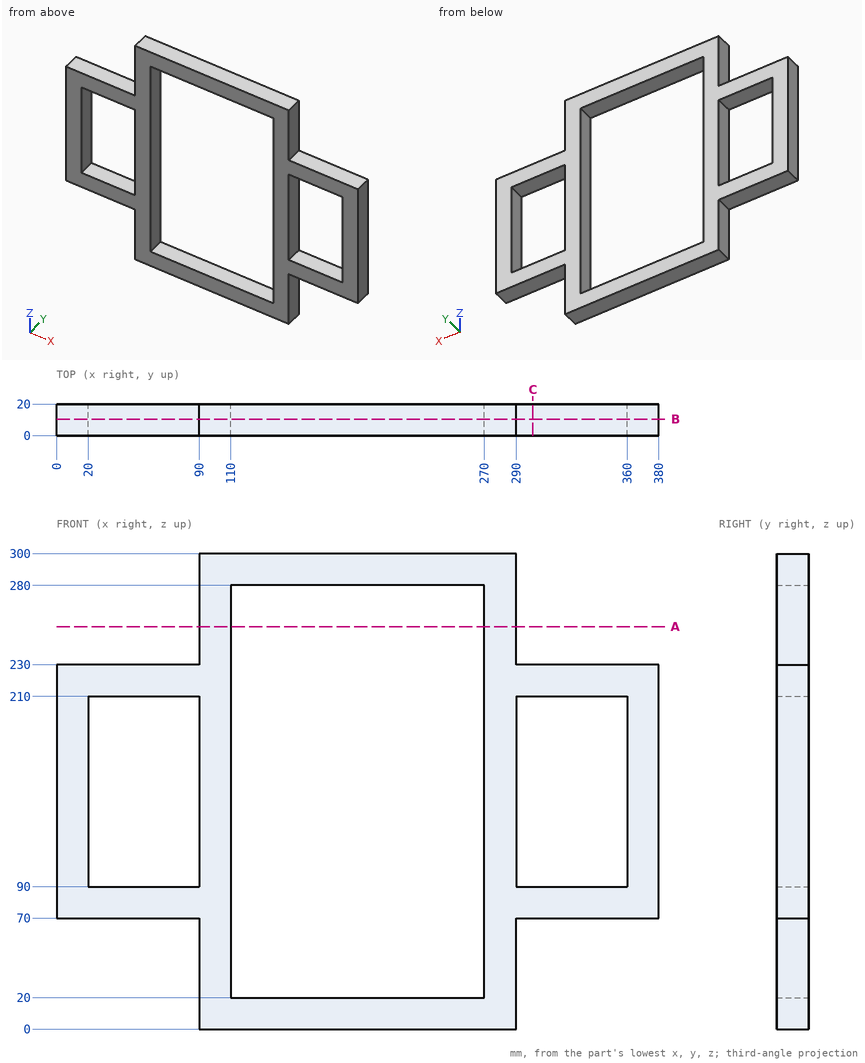
Drawing for the job (mm, zero at the part's lowest x, y, z). Round coordinates to 2 decimals unless told otherwise and drop trailing zeros. Write each loop counter-clockwise with the first axis right and the second up, starting at its lowest first coordinate (ties: lowest second). Pieces come first, ordered by that corner, then holes.
Item 1: Band-saw the part on B-B on y = 10.5. Write the cut outline in (x, z), then the cut area to 3 significant figures.
Filled in:
outline: (0, 70) - (90, 70) - (90, 0) - (290, 0) - (290, 70) - (380, 70) - (380, 230) - (290, 230) - (290, 300) - (90, 300) - (90, 230) - (0, 230) - close; hole (20, 90) - (90, 90) - (90, 210) - (20, 210) - close; hole (110, 20) - (270, 20) - (270, 280) - (110, 280) - close; hole (290, 90) - (360, 90) - (360, 210) - (290, 210) - close
area: 30,400 mm2
Item 2: Band-saw the part on A-A on z = 254. Write the cut outline in (x, y), then the cut area to 3 significant figures.
Filled in:
outline: (90, 0) - (110, 0) - (110, 20) - (90, 20) - close; (270, 0) - (290, 0) - (290, 20) - (270, 20) - close
area: 800 mm2
Item 3: Drop flat-ended pins along their axis: pin 1 Ø6 at (x, y) = (337.5, 12.5) entering from -Z; pin 2 Ø6 at (y, z) = (12.5, 38) entering from -X; pin 3 Ø6 at (x, y) = (61.5, 8.5) entering from +Z. Give the stop position or say it passes through.
Filled in:
pin 1: stops at z = 70
pin 2: stops at x = 90
pin 3: stops at z = 230
Item 4: Drill centre lines: L1, parallel to X at y = 4.5, z = 186; L2, parallel to Z at x = 328.5, y = 6.75; L3, parallel to X at y = 19, z = 239.5. Where is each one in solid material? Low to high.
Filled in:
L1: x = 0 to 20, 90 to 110, 270 to 290, 360 to 380
L2: z = 70 to 90, 210 to 230
L3: x = 90 to 110, 270 to 290
Item 5: Band-saw the part on C-C on x = 300.5. Write the cut outline in (y, z), then the cut area to 3 significant figures.
Filled in:
outline: (0, 70) - (20, 70) - (20, 90) - (0, 90) - close; (0, 210) - (20, 210) - (20, 230) - (0, 230) - close
area: 800 mm2
